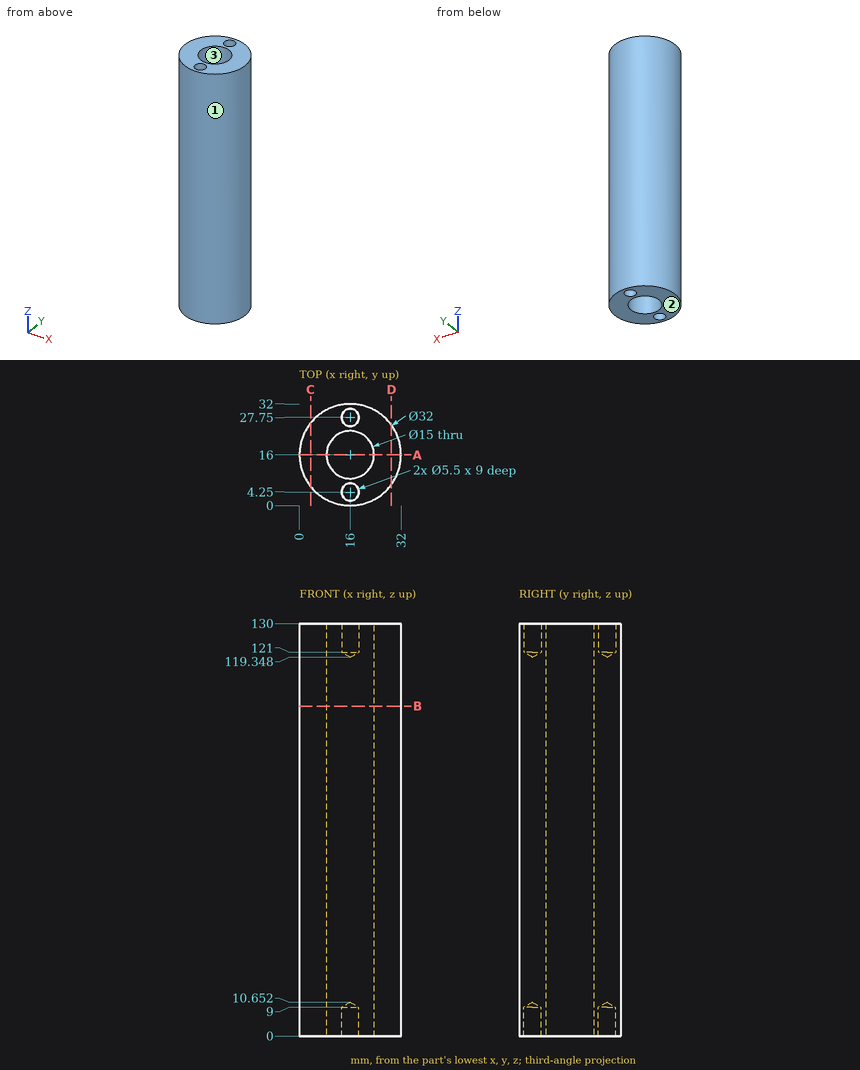
For this review, use the dimensioned drawing (mm, ordinates from the lowest corner) and the shaded views. Round coordinates to 2 decimals unless told otherwise and drop trailing zeros. Write each loop counter-clockwise with the first axis right and the second up, starting at its lowest first coordinate (ties: lowest second). Pieces come first, ordered by that corner, then holes. Notation, with made-up numbers: (-33, -4) -> (26, -4) arc R5 cw to (26, 4) -> close; hole circle Ø7 at (53, 40.25). An arc over 180 degrees is marked (long way). Use CSV: the item, a comma, the result in double quotes.
Q1. For pin 1 Ø12 at (y, z) = (5, 81) entering from -X; pin 2 Ø5 at (x, y) = (16, 4.25) entering from +Z; pin 3 Ø1 at (x, z) = (20, 56) entering from -Y, all flat-tipped, find the tip position at first contact; note any pin that passes through.
Checks:
pin 1,"x = 0.8"
pin 2,"z = 120.85"
pin 3,"y = 0.39"
Q2. To check wall thickness, follow probe 1 along Y at (x, z) = (16, 123.5); probe 2 along X at (y, z) = (15, 24.5); probe 3 along X at (y, z) = (18.5, 16). State the ranges of each line that lie inside material, in increasing order. Write a range as [from, to].
Checks:
probe 1,"[0, 1.5], [7, 8.5], [23.5, 25], [30.5, 32]"
probe 2,"[0.03, 8.57], [23.43, 31.97]"
probe 3,"[0.2, 8.93], [23.07, 31.8]"
Q3. Consider section B-B (z = 104). Give the boundary of the cut face in (x, y).
Checks:
outline,"circle Ø32 at (16, 16); hole circle Ø15 at (16, 16)"
Q4. Mouldability with a two-part tool opening along Y and no side actions: class the marked faces 1, 2 and 3 as released by +Y, released by -Y, zero draft, split by the parting line, or undercut.
Checks:
face 1,"split by the parting line"
face 2,"zero draft"
face 3,"undercut"
Q5. Consider section D-D (x = 29). Give the boundary of the cut face in (y, z), then the cut area to 4 significant figures.
Checks:
outline,"(6.67, 0) -> (25.33, 0) -> (25.33, 130) -> (6.67, 130) -> close"
area,"2,425 mm²"
Q6. Consider section C-C (x = 3.5). Give the boundary of the cut face in (y, z).
Checks:
outline,"(6.01, 0) -> (25.99, 0) -> (25.99, 130) -> (6.01, 130) -> close"
Q7. Consider section A-A (y = 16). Give the boundary of the cut face in (x, z).
Checks:
outline,"(0, 0) -> (8.5, 0) -> (8.5, 130) -> (0, 130) -> close; (23.5, 0) -> (32, 0) -> (32, 130) -> (23.5, 130) -> close"
